```python
from build123d import *

# Parameters (mm, degrees)
SKETCH_1_W      = 60
SKETCH_1_H      = 20
SKETCH_1_R      = 2.2
EXTRUDE_1_DEPTH = 6.25
FILLET_1_R      = 3


with BuildPart() as part:
    # 草图1 → 凸台-拉伸1 (new, symmetric)
    with BuildSketch(Plane(origin=(0, 0, 0), x_dir=(1, 0, 0), z_dir=(0, 1, 0))):
        Rectangle(SKETCH_1_W, SKETCH_1_H)
        with Locations(Location((0, 0, 0), (0, 0, 270))):
            Circle(SKETCH_1_R, mode=Mode.SUBTRACT)
        with Locations(Location((-20, 0, 0), (0, 0, 270))):
            Circle(SKETCH_1_R, mode=Mode.SUBTRACT)
        with Locations(Location((20, 0, 0), (0, 0, 90))):
            Circle(SKETCH_1_R, mode=Mode.SUBTRACT)
    extrude(amount=EXTRUDE_1_DEPTH, both=True)

    # 圆角1
    fillet_1_edges = [part.edges().sort_by_distance(p)[0] for p in [
        (30, 0, 10),
        (-30, 0, 10),
        (-30, 0, -10),
        (30, 0, -10),
    ]]
    fillet(fillet_1_edges, radius=FILLET_1_R)


solid = part.part
```
The listing builds one solid part. Answer for the finished solid, in the listing's coordinates (mm). Coordinates: 2 decimals unless noted, no trailing zeros. Write each loop counter-clockwise with the first axis right and the second up, starting at its lowest first coordinate (ties: lowest second). Pieces come first, ordered by that corner, then holes. Notation, with made-up numbers: (24.25, -37.5) - (82.25, -37.5) arc R9 ccw to (82.25, -30.5) - close; hole circle Ø10 at (72.25, -38). An arc over 180 degrees is marked (long way). Return JSON: item names as keys, results as strings. Group by question number.
Q1. The part is cut by section B-B on x = 0. Write down the section's boundary in (y, z).
Q2. The part is cut by section A-A on y = -4.75. Write down the section's boundary in (x, z).
Q3. A flat-ended cylindrical pin translates along its axis: pin 1 Ø4 at (x, z) = (18, 0) entering from -Y. Find the tip coordinate at first contact, or state that the pin passes through.
Q4. The part is cut by section D-D on x = 19. Write down the section's boundary in (y, z).
Q5. For a pull along Z with two mould halves and no side action, classify faces 1 (the cylindrical face through (-29.14, -0.09, -9.1)), 2 (the cylindrical face through (-22.148, -0.088, -0.477)), 3 (the flat face through (-0.4, -6.25, -2.4)) as +Z half, -Z half, draft (parallel to the pull), parting line (faces both ways), or undercut.
Q6. The part is cut by section C-C on z = 0. Write down the section's boundary in (x, y), and give its area (3 significant figures).
Q7. Find the intervals of material crossed by line 1 along X through (y, z) = (-3.25, 0); line 2 along Z through (x, y) = (20, -3); line 3 along X through (y, z) = (0.5, -7.25), in increasing order. Write a range as [from, to].
Evaluation:
{
 "1": {"outline": "(-6.25, -10) - (6.25, -10) - (6.25, -2.2) - (-6.25, -2.2) - close; (-6.25, 2.2) - (6.25, 2.2) - (6.25, 10) - (-6.25, 10) - close"},
 "2": {"outline": "(-30, -7) arc R3 ccw to (-27, -10) - (27, -10) arc R3 ccw to (30, -7) - (30, 7) arc R3 ccw to (27, 10) - (-27, 10) arc R3 ccw to (-30, 7) - close; hole circle Ø4.4 at (-20, 0); hole circle Ø4.4 at (0, 0); hole circle Ø4.4 at (20, 0)"},
 "3": {"pin 1": "stops at y = -6.25"},
 "4": {"outline": "(-6.25, -10) - (6.25, -10) - (6.25, -1.96) - (-6.25, -1.96) - close; (-6.25, 1.96) - (6.25, 1.96) - (6.25, 10) - (-6.25, 10) - close"},
 "5": {"face 1": "-Z half", "face 2": "undercut", "face 3": "draft"},
 "6": {"outline": "(-30, -6.25) - (-22.2, -6.25) - (-22.2, 6.25) - (-30, 6.25) - close; (-17.8, -6.25) - (-2.2, -6.25) - (-2.2, 6.25) - (-17.8, 6.25) - close; (2.2, -6.25) - (17.8, -6.25) - (17.8, 6.25) - (2.2, 6.25) - close; (22.2, -6.25) - (30, -6.25) - (30, 6.25) - (22.2, 6.25) - close", "area": "585 mm2"},
 "7": {"line 1": "x = [-30, -22.2], [-17.8, -2.2], [2.2, 17.8], [22.2, 30]", "line 2": "z = [-10, -2.2], [2.2, 10]", "line 3": "x = [-29.99, 29.99]"}
}
